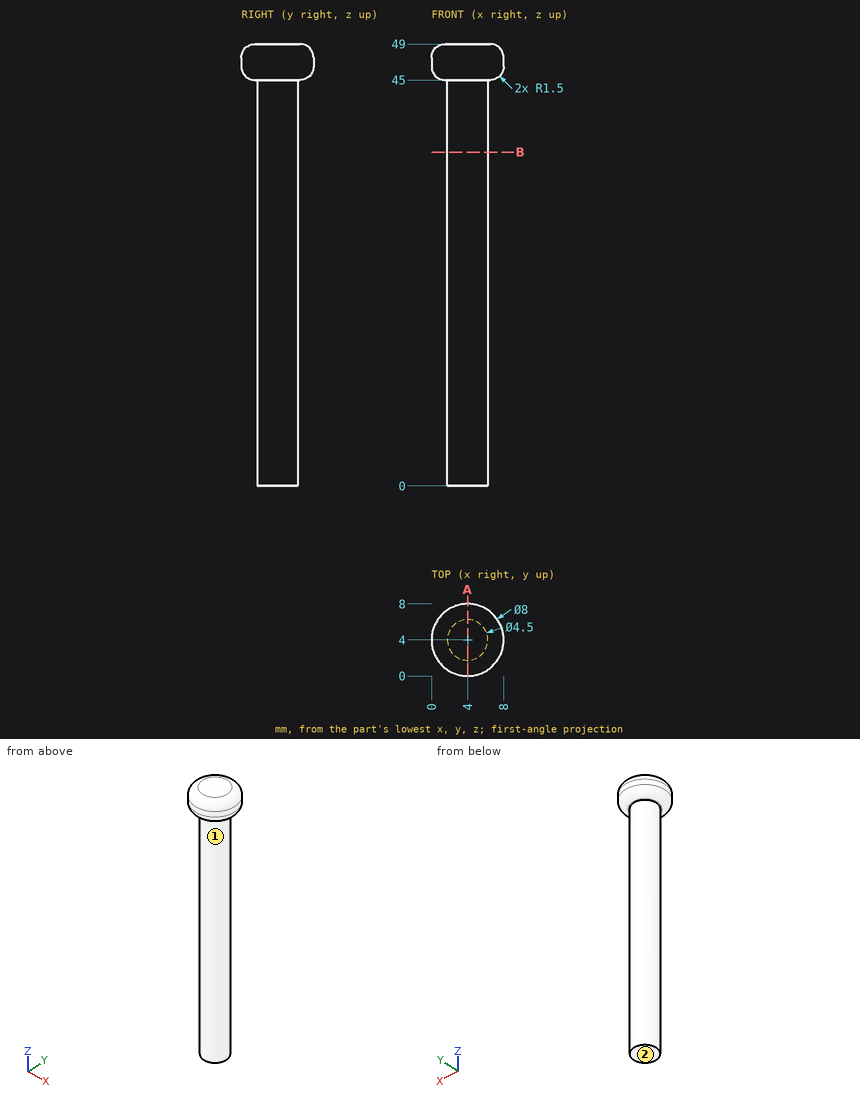
The drawing under review shows one solid part. Ordinate dimensions are in mm from its lowest x, y, z. A direction names the side the tool comes from. Round coordinates to 2 decimals unless told otherwise and drop trailing zeros. Loops run counter-clockwise (first coordinate to the right, second up) from the corner with the lowest first, then second, coordinate; pieces in that order, holes last. Notation, with made-up numbers: M -23,57 L -11,57 A24 cw -11,83 Z; hole C 52.5,44.25 d4. An arc over 180 degrees is marked long. Answer as CSV lines item,"result". Start each with the question number.
Item 1: Insertion check: P1, Ø3, axis at x = 2.5, z = 27, coming from the -Y side; P2, Ø2, axis at x = 5.5, z = 14.5, coming from the +Y side; P3, Ø4, axis at y = 1, z = 31, coming from the +X side. Each pin has a flat end and moves straight along its axis. Give the tip position at first contact, or say it passes through.
Item 2: Wall thickness on line 1 (Y direction, x = 2.5, z = 19); line 2 (Y direction, x = 5.25, z = 18): over which ranges is each line inside the solid? List them lowest first. Write a range as [from, to].
Item 3: For the marked faces 1 and 2, list the 3-axis set-ups (+Z, -Z, +X, -X, +Y, -Y) from which the entire face can be reached by the end or side of a thin tool; tool diameter is ignored.
Item 4: Consider section A-A (x = 4). Write out the cut boundary in (y, z).
Item 5: Consider section B-B (z = 37). Write out the cut boundary in (x, y), then the cut area to 3 significant figures.
Answer:
1,P1,"stops at y = 1.75"
1,P2,"stops at y = 6.19"
1,P3,"stops at x = 6.02"
2,line 1,"y = [2.32, 5.68]"
2,line 2,"y = [2.13, 5.87]"
3,face 1,"-Z"
3,face 2,"-Z, +X, -X, +Y, -Y"
4,outline,"M 0,46.5 A1.5 ccw 1.5,45 L 1.75,45 L 1.75,0 L 6.25,0 L 6.25,45 L 6.5,45 A1.5 ccw 8,46.5 L 8,47.5 A1.5 ccw 6.5,49 L 1.5,49 A1.5 ccw 0,47.5 Z"
5,outline,"C 4,4 d4.5"
5,area,"15.9 mm^2"
